Job drawing, mm, ordinate dimensions from the low corner. One solid piece. Coordinates: 2 decimals unless noted, no trailing zeros. Write each loop counter-clockwise with the first axis right and the second up, starting at its lowest first coordinate (ties: lowest second). Pieces come first, ordered by that corner, then holes. Notation, with made-up numbers: M -33,55.25 L 14,55.25 A14 cw 14,67.25 Z; hole C 43.5,23.25 d2. An arc over 180 degrees is marked long. Answer as CSV lines item,"result". Start each with the question number.
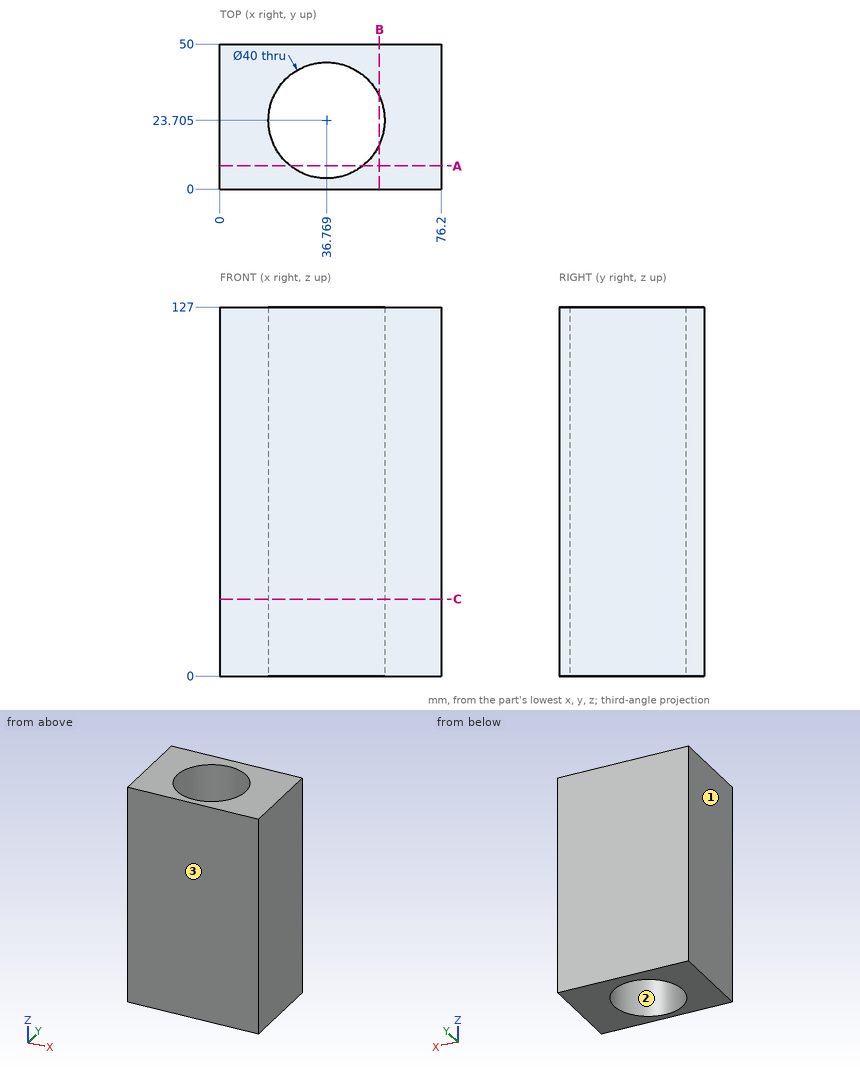
1) Band-saw the part on C-C, the plane z = 26.5. List the corners of the cut face in (x, y) (1 decimal).
2) Band-saw the part on B-B, the plane x = 55. List the corners of the cut face in (y, z), plus the area to 3 significant figures.
3) Probe L1, parallel to X at y = 28, z = 59.5 (1 decimal); L2, parallel to X at y = 35.5, z = 35; L3, parallel to Y at x = 34, z = 10. List the from-to ranges inside material, lowest first. Write a range as [from, to].
4) Two-plate mould, pull along Y, no slides. Class the marked faces 1, 2 and 3: pulls with the +Y half, pulls with the -Y half, needs draft (parallel to the pull), parting line crosses it, or undercut.
5) Band-saw the part on A-A, the plane y = 8. List the corners of the cut face in (x, z) (1 decimal), plus the area to 3 significant figures.
Result sheet:
1,outline,"M 0,0 L 76.2,0 L 76.2,50 L 0,50 Z; hole C 36.8,23.7 d40"
2,outline,"M 0,0 L 15.48,0 L 15.48,127 L 0,127 Z; M 31.93,0 L 50,0 L 50,127 L 31.93,127 Z"
2,area,"4,260 mm²"
3,L1,"x = [0, 17.2], [56.3, 76.2]"
3,L2,"x = [0, 20.62], [52.92, 76.2]"
3,L3,"y = [0, 3.9], [43.51, 50]"
4,face 1,"needs draft"
4,face 2,"undercut"
4,face 3,"pulls with the -Y half"
5,outline,"M 0,0 L 24.4,0 L 24.4,127 L 0,127 Z; M 49.2,0 L 76.2,0 L 76.2,127 L 49.2,127 Z"
5,area,"6,530 mm²"
